Here's how the part is built. I have some questions about the finished solid (model axes, mm). Face numbers are marked on the shaded views. A direction names the side the tool comes from. Coordinates: 2 decimals unless noted, no trailing zeros. Loops run counter-clockwise (first coordinate to the right, second up) from the corner with the lowest first, then second, coordinate; pieces in that order, holes last. Notation, with made-up numbers: M 3.25,2 L 29.25,2 A22 ccw 29.25,25 Z; hole C -10.75,18.5 d10. An arc over 180 degrees is marked long. Use one line per item in the form item = value. Start each with the question number.
(1) Imagine slicing it at D-D, the plane z = -17.75. Please give me the cut outline in (x, y).
(2) Will this pin go through, and if not, where does the flat tip stop? P1, Ø2.5, axis at x = 77.86, z = -3, coming from the +Y side.
(3) Thinking about a two-plate mould opening in Z: for the marked faces 1, 2 and 3, which applies, +Z half, -Z half, draft (parallel to the pull), parting line (faces both ways), or undercut?
(4) Imagine slicing it at B-B, the plane x = 57. Please give me the cut outline in (y, z).
(5) Imagine slicing it at A-A, the plane x = 3. Please give me the cut outline in (y, z).
(6) On a 3-axis mill with a long thin cutter (end or side, diameter ignored), from which of +Z, -Z, +X, -X, +Y, -Y can I reach the whole of each face in a straight line? I mean the marked faces 4 and 5. Say none if no direction works.
(7) Please list where these lines run through material, in increasing order: L1, parallel to Z at x = 60.5, y = 1.2; L2, parallel to Z at x = 66, y = 1.2; L3, parallel to X at y = 5.1, z = -2.5.
(8) Imagine slicing it at C-C, the plane z = -5.5. Please give me the cut outline in (x, y), and give its area (3 significant figures).
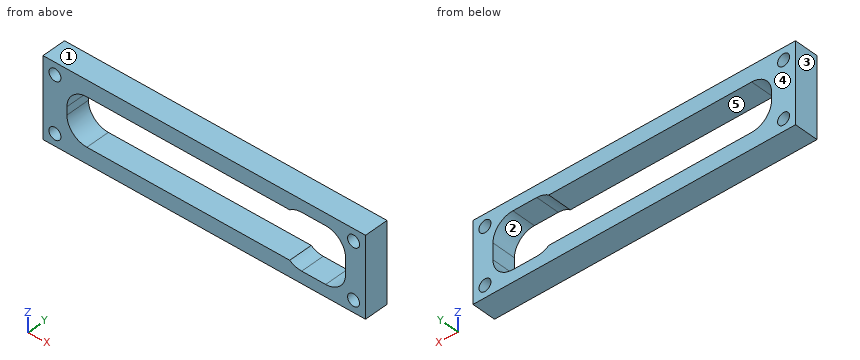
```python
from build123d import *

# Parameters (mm, degrees)
SKETCH1_W           = 80.863890266
SKETCH1_H           = 20
SKETCH1_R           = 1.5
SKETCH1_W_2         = 68.863890266
SKETCH1_H_2         = 12
BOSS_EXTRUDE1_DEPTH = 6
CUT_EXTRUDE1_DEPTH  = 84.516278347
FILLET1_R           = 5


with BuildPart() as part:
    # Sketch1 → Boss-Extrude1 (new body)
    with BuildSketch(Plane(origin=(0, 0, 0), x_dir=(1, 0, 0), z_dir=(0, 1, 0))):
        with Locations((40.431945133, 10)):
            Rectangle(SKETCH1_W, SKETCH1_H)
        with Locations(Location((3, 17, 0), (0, 0, 270))):
            Circle(SKETCH1_R, mode=Mode.SUBTRACT)
        with Locations(Location((3, 3, 0), (0, 0, 90))):
            Circle(SKETCH1_R, mode=Mode.SUBTRACT)
        with Locations(Location((77.863890266, 3, 0), (0, 0, 270))):
            Circle(SKETCH1_R, mode=Mode.SUBTRACT)
        with Locations(Location((77.863890266, 17, 0), (0, 0, 90))):
            Circle(SKETCH1_R, mode=Mode.SUBTRACT)
        with Locations((40.431945133, 10)):
            Rectangle(SKETCH1_W_2, SKETCH1_H_2, mode=Mode.SUBTRACT)
    extrude(amount=BOSS_EXTRUDE1_DEPTH)

    # Sketch2 → Cut-Extrude1 (cut, through all)
    with BuildSketch(Plane(origin=(0, 6, 0), x_dir=(1, 0, 0), z_dir=(0, 1, 0))):
        Polygon((61.863890266, 17), (61.863890266, 16), (74.863890266, 16), (74.863890266, 4), (61.863890266, 4), (61.863890266, 3), (75.863890266, 3), (75.863890266, 17), align=None)
    extrude(amount=-CUT_EXTRUDE1_DEPTH, mode=Mode.SUBTRACT)

    # Fillet1
    # the kernel refuses this fillet: 5 mm, written as the material it adds along each edge
    with BuildSketch(Plane(origin=(75.863890266, 6, -17), x_dir=(0, 0, 1), z_dir=(0, -1, 0)), Plane(origin=(75.863890266, 6, -3), x_dir=(-1, 0, 0), z_dir=(0, -1, 0)), Plane(origin=(6, 0, -16), x_dir=(0, 0, 1), z_dir=(0, 1, 0))) as fillet1_piece_1:
        with BuildLine():
            CenterArc((FILLET1_R, FILLET1_R), FILLET1_R, 180, 90)
            Line((0, FILLET1_R), (-FILLET1_R * 0.02, FILLET1_R))
            Line((-FILLET1_R * 0.02, FILLET1_R), (-FILLET1_R * 0.02, -FILLET1_R * 0.02))
            Line((-FILLET1_R * 0.02, -FILLET1_R * 0.02), (FILLET1_R, -FILLET1_R * 0.02))
            Line((FILLET1_R, -FILLET1_R * 0.02), (FILLET1_R, 0))
        make_face()
    extrude(amount=6)
    with BuildSketch(Plane(origin=(61.863890266, 6, -17), x_dir=(1, 0, 0), z_dir=(0, -1, 0))) as fillet1_piece_2:
        with BuildLine():
            CenterArc((3, 5), FILLET1_R, 233.130102354, 36.869897646)
            Line((0, 1), (-0.06, 0.92))
            ThreePointArc((-0.06, 0.92), (-0.1, 0.5), (-0.1, 0))
            Line((-0.1, 0), (0, -0.1))
            Line((0, -0.1), (3, -0.1))
            Line((3, -0.1), (3, 0))
        make_face()
    extrude(amount=6)
    with BuildSketch(Plane(origin=(61.863890266, 6, -3), x_dir=(0, 0, -1), z_dir=(0, -1, 0))) as fillet1_piece_3:
        with BuildLine():
            CenterArc((5, 3), FILLET1_R, 180, 36.869897646)
            Line((0, 3), (-0.1, 3))
            Line((-0.1, 3), (-0.1, 0))
            Line((-0.1, 0), (0, -0.1))
            ThreePointArc((0, -0.1), (0.5, -0.1), (0.92, -0.06))
            Line((0.92, -0.06), (1, 0))
        make_face()
    extrude(amount=6)
    with BuildSketch(Plane(origin=(6, 0, -4), x_dir=(0, 0, -1), z_dir=(0, 1, 0))) as fillet1_piece_4:
        with BuildLine():
            CenterArc((FILLET1_R, -FILLET1_R), FILLET1_R, 90, 90)
            Line((0, -FILLET1_R), (-FILLET1_R * 0.02, -FILLET1_R))
            Line((-FILLET1_R * 0.02, -FILLET1_R), (-FILLET1_R * 0.02, FILLET1_R * 0.02))
            Line((-FILLET1_R * 0.02, FILLET1_R * 0.02), (FILLET1_R, FILLET1_R * 0.02))
            Line((FILLET1_R, FILLET1_R * 0.02), (FILLET1_R, 0))
        make_face()
    extrude(amount=6)


solid = part.part
```
Answer:
q1.outline = M 0,0 L 1.7,0 L 1.7,6 L 0,6 Z; M 4.3,0 L 76.56,0 L 76.56,6 L 4.3,6 Z; M 79.16,0 L 80.86,0 L 80.86,6 L 79.16,6 Z
q2.P1 = through
q3.face_1 = +Z half
q3.face_2 = undercut
q3.face_3 = draft
q4.outline = M 0,-20 L 6,-20 L 6,-16 L 0,-16 Z; M 0,-4 L 6,-4 L 6,0 L 0,0 Z
q5.outline = M 0,-20 L 6,-20 L 6,-18.5 L 0,-18.5 Z; M 0,-15.5 L 6,-15.5 L 6,-4.5 L 0,-4.5 Z; M 0,-1.5 L 6,-1.5 L 6,0 L 0,0 Z
q6.face_4 = +Z, -Z, +X, -X, +Y
q6.face_5 = +Y, -Y
q7.L1 = -20 to -16, -4 to 0
q7.L2 = -20 to -17, -3 to 0
q7.L3 = 0 to 1.59, 4.41 to 76.45, 79.28 to 80.86
q8.outline = M 0,0 L 7.43,0 L 7.43,6 L 0,6 Z; M 75.19,0 L 80.86,0 L 80.86,6 L 75.19,6 Z
q8.area = 78.6 mm²
